Autodesk Inventor part; units mm, degrees
ref_plane "YZ Plane" through (0, 0, 0) normal (1, 0, 0) x (0, 1, 0)
ref_plane "XZ Plane" through (0, 0, 0) normal (0, 1, 0) x (-1, 0, 0)
ref_plane "XY Plane" through (0, 0, 0) normal (0, 0, 1) x (1, 0, 0)
sketch "Sketch1" plane through (0, 0, 0) normal (0, 0, 1) x (1, 0, 0)
  circle A0 centre (0, 0) radius 17.526
  dimension "d0" = 35.052
extrude "Extrusion1" add sketch "Sketch1" along normal blind 1.5875
sketch "Sketch2" plane through (0, 0, 1.5875) normal (0, 0, 1) x (1, 0, 0)
  circle A0 centre (0, 0) radius 12.7
  dimension "d3" = 25.4
extrude "Extrusion2" add sketch "Sketch2" along normal blind 9.525
sketch "Sketch3" plane through (0, 0, 0) normal (0, 0, -1) x (-1, 0, 0)
  circle A0 centre (0, 0) radius 7.3787
  dimension "d6" = 14.7574
extrude "Extrusion3" add sketch "Sketch3" along normal blind 1.5875
sketch "Sketch4" plane through (0, 0, -1.5875) normal (0, 0, -1) x (-1, 0, 0)
  circle A0 centre (0, 0) radius 3.5687
  dimension "d9" = 7.1374
extrude "Extrusion4" add sketch "Sketch4" along normal blind 3.175
sketch "Sketch5" plane through (0, 0, 11.1125) normal (0, 0, 1) x (1, 0, 0)
  circle A0 centre (0, 0) radius 1.524
  dimension "d12" = 3.048
extrude "Extrusion5" add sketch "Sketch5" along normal blind 3.175
properties part number "Wheel"
The model under review builds one solid part; all positions refer to its coordinate system, in mm. A direction names the side the tool comes from. Give positions to 0.01 mm unless a question says otherwise; leave off trailing zeros. Write each loop counter-clockwise with the first axis right and the second up, starting at its lowest first coordinate (ties: lowest second). Pieces come first, ordered by that corner, then holes.
(1) Consider section D-D, the plane y = 9. Give the boundary of the cut face in (x, z), and give its area (3 significant figures).
(2) Tool access review of faces 1 (the cylindrical face through (-2.75, 12.4, 6.28)), 2 (the cylindrical face through (-7.038, -2.216, -0.783)), 3 (the flat face through (0, 0, -4.762)): name each direction out of +Z, -Z, +X, -X, +Y, -Y from which nothing blocks a thin tool from reaching the whole face with its end or side.
(3) Consider section C-C, the plane z = 7. Give the boundary of the cut face in (x, y).
(4) To check wall thickness, follow L1, parallel to Z at x = -9, y = 11; L2, parallel to Z at x = 10.5, y = 7; L3, parallel to X at y = 1, z = -2.5. State the ranges of each line that lie inside material, in increasing order.
(5) For P1, Ø6, axis at y = 3.5, z = 10, coming from the -X side; P2, Ø1.5, axis at x = 8, y = 6.5, coming from the +Z side; P3, Ø1.5, axis at x = 4.5, z = 3.5, coming from the -Y side, all flat-tipped, find the tip position at first contact; note any pin that passes through.
(6) Consider section A-A, the plane x = 0. Give the boundary of the cut face in (y, z), and give its area (3 significant figures).
Returned:
1. outline: (-15.04, 0) - (15.04, 0) - (15.04, 1.59) - (8.96, 1.59) - (8.96, 11.11) - (-8.96, 11.11) - (-8.96, 1.59) - (-15.04, 1.59) - close
1. area: 218 mm2
2. face 1: +Z
2. face 2: -Z
2. face 3: -Z, +X, -X, +Y, -Y
3. outline: circle Ø25.4 at (0, 0)
4. L1: z = 0 to 1.59
4. L2: z = 0 to 11.11
4. L3: x = -3.43 to 3.43
5. P1: stops at x = -12.69
5. P2: stops at z = 11.11
5. P3: stops at y = -12.13
6. outline: (-17.53, 0) - (-7.38, 0) - (-7.38, -1.59) - (-3.57, -1.59) - (-3.57, -4.76) - (3.57, -4.76) - (3.57, -1.59) - (7.38, -1.59) - (7.38, 0) - (17.53, 0) - (17.53, 1.59) - (12.7, 1.59) - (12.7, 11.11) - (1.52, 11.11) - (1.52, 14.29) - (-1.52, 14.29) - (-1.52, 11.11) - (-12.7, 11.11) - (-12.7, 1.59) - (-17.53, 1.59) - close
6. area: 353 mm2
